Model file for the job. Use its own axes, mm. Face numbers are marked on the shaded views. A direction names the side the tool comes from. Coordinates: 2 decimals unless noted, no trailing zeros. Write each loop counter-clockwise with the first axis right and the second up, starting at its lowest first coordinate (ties: lowest second). Pieces come first, ordered by that corner, then holes. Notation, with made-up numbers: (-32.75, -40) -> (-6.75, -40) arc R33 ccw to (-6.75, -5) -> close; hole circle Ø11 at (-35, 79.25). An arc over 180 degrees is marked (long way). Write item = value, one per line. Start each with the question number.
from build123d import *

# Parameters (mm, degrees)
PAD_DEPTH       = 1.7
SKETCH001_W     = 8.9
SKETCH001_H     = 14.15
PAD010_DEPTH    = 10.82
SKETCH021_R     = 3.185
SKETCH021_R_2   = 1
POCKET010_DEPTH = 10
FILLET014_R     = 1


with BuildPart() as part:
    # Sketch → Pad (new body)
    with BuildSketch(Plane.XY):
        with BuildLine():
            Line((0, 0), (30, 0))
            Line((30, 0), (30, 1))
            Line((30, 1), (31, 1))
            Line((31, 1), (31, 18.27))
            Line((31, 18.27), (24.4, 18.27))
            ThreePointArc((24.4, 24.87), (21.1, 21.57), (24.4, 18.27))
            Line((24.4, 24.87), (31, 24.87))
            Line((31, 24.87), (31, 59.13))
            Line((31, 59.13), (24.4, 59.13))
            ThreePointArc((24.4, 65.73), (21.1, 62.43), (24.4, 59.13))
            Line((24.4, 65.73), (31, 65.73))
            Line((31, 65.73), (31, 83))
            Line((30, 83), (31, 83))
            Line((30, 84), (30, 83))
            Line((30, 84), (0, 84))
            Line((0, 84), (-30, 84))
            Line((-30, 84), (-30, 83))
            Line((-30, 83), (-31, 83))
            Line((-31, 83), (-31, 65.73))
            Line((-31, 65.73), (-24.4, 65.73))
            ThreePointArc((-24.4, 59.13), (-21.1, 62.43), (-24.4, 65.73))
            Line((-24.4, 59.13), (-31, 59.13))
            Line((-31, 59.13), (-31, 24.87))
            Line((-31, 24.87), (-24.4, 24.87))
            ThreePointArc((-24.4, 18.27), (-21.1, 21.57), (-24.4, 24.87))
            Line((-24.4, 18.27), (-31, 18.27))
            Line((-31, 18.27), (-31, 1))
            Line((-31, 1), (-30, 1))
            Line((-30, 1), (-30, 0))
            Line((-30, 0), (0, 0))
        make_face()
    extrude(amount=PAD_DEPTH)

    # Sketch001 → Pad010 (new body)
    with BuildSketch(Plane.XY.offset(1.7)):
        with Locations((-22.74, 80.955)):
            Rectangle(SKETCH001_W, SKETCH001_H)
    extrude(amount=PAD010_DEPTH)

    # Sketch021 → Pocket010 (cut)
    with BuildSketch(Plane(origin=(0, 88.03, 0), x_dir=(-1, 0, 0), z_dir=(0, 1, 0))):
        with Locations((22.74, 8.02)):
            Circle(SKETCH021_R)
        with Locations((22.74, 8.02)):
            Circle(SKETCH021_R_2, mode=Mode.SUBTRACT)
    extrude(amount=-POCKET010_DEPTH, mode=Mode.SUBTRACT)

    # Fillet014
    fillet014_edges = [part.edges().sort_by_distance(p)[0] for p in [
        (-21.74, 88.03, 8.02),
    ]]
    fillet(fillet014_edges, radius=FILLET014_R)


solid = part.part
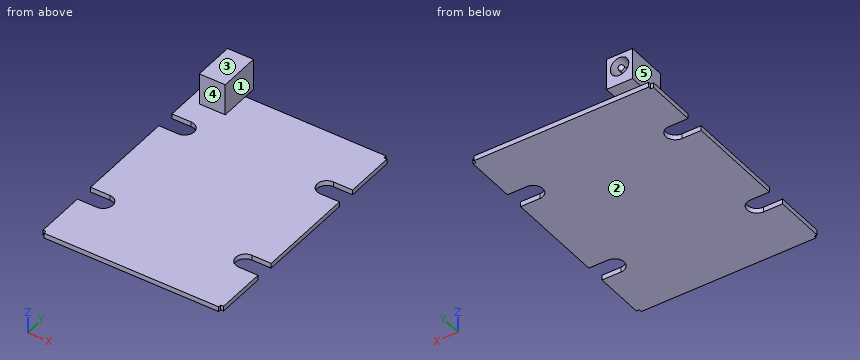
(1) Saw through at B-B (z = 8.02). Give the cut face in (x, y) (3 decimals).
(2) 3-axis set-ups, long thin cutter, end or side, ignore diameter. For the marked faces 1, 2, 3, 4 and 5: which of +Z, -Z, +X, -X, +Y, -Y reach the whole face in a straight line?
(3) Saw through at C-C (y = 41). Give the cut face in (x, z).
(4) Saw through at D-D (x = -13.5). Give the cut face in (y, z).
(5) Saw through at A-A (x = 27). Give the cut face in (y, z).
(6) Drill centre lines: line 1 along Y through (x, z) = (-25, 1.25); line 2 along Z through (x, y) = (-22.74, 82.75) (3 decimals); line 3 along X through (y, z) = (80, 5.25). Where is each one in solid material? Low to high.
(7) Drop flat-ended pins along their axis: pin 1 Ø1.4 at (x, z) = (-29, 1) entering from +Y; pin 2 Ø0.8 at (y, z) = (0.5, 1) entering from +X; pin 3 Ø2 at (x, z) = (-19.5, 6.5) entering from -Y; pin 4 Ø1.5 at (y, z) = (71.5, 11) entering from +X. Give the stop position or say it passes through.
Returned:
q1.outline = (-27.19, 73.88) -> (-18.29, 73.88) -> (-18.29, 88.03) -> (-19.555, 88.03) -> (-19.555, 78.03) -> (-21.74, 78.03) -> (-21.74, 87.03) arc R1 ccw to (-23.74, 87.03) -> (-23.74, 78.03) -> (-25.925, 78.03) -> (-25.925, 88.03) -> (-27.19, 88.03) -> close
q2.face_1 = +Z, +X, +Y, -Y
q2.face_2 = -Z, +X, -X, +Y, -Y
q2.face_3 = +Z, +X, -X, +Y, -Y
q2.face_4 = +Z, +X, -X, -Y
q2.face_5 = +Z, -X, +Y, -Y
q3.outline = (-31, 0) -> (31, 0) -> (31, 1.7) -> (-31, 1.7) -> close
q4.outline = (0, 0) -> (84, 0) -> (84, 1.7) -> (0, 1.7) -> close
q5.outline = (0, 0) -> (18.27, 0) -> (18.27, 1.7) -> (0, 1.7) -> close; (24.87, 0) -> (59.13, 0) -> (59.13, 1.7) -> (24.87, 1.7) -> close; (65.73, 0) -> (84, 0) -> (84, 1.7) -> (65.73, 1.7) -> close
q6.line_1 = 0 to 18.27, 24.87 to 59.13, 65.73 to 84
q6.line_2 = 0 to 4.835, 7.02 to 9.02, 11.205 to 12.52
q6.line_3 = -27.19 to -24.31, -21.17 to -18.29
q7.pin_1 = 84
q7.pin_2 = 30
q7.pin_3 = 73.88
q7.pin_4 = through
